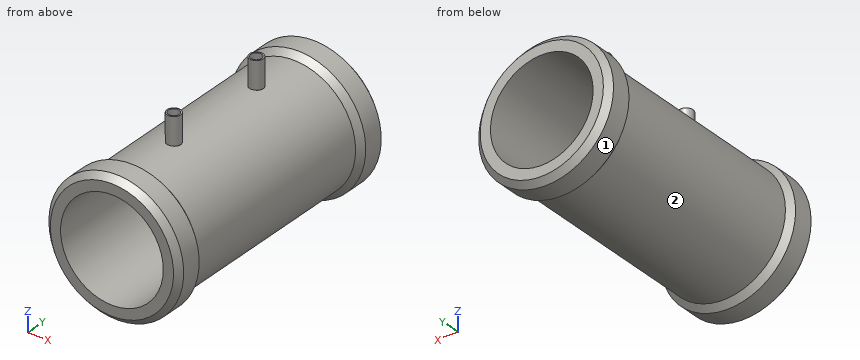
```python
from build123d import *

# Parameters (mm, degrees)
F0_R          = 45
F0_R_2        = 37.5
F1_DEPTH      = 100
F3_R          = 5
F3_R_2        = 4
F4_DEPTH      = 20
F4_DEPTH_BACK = 5


# Not quite as in the source:
# - a pattern or mirror of a feature is missing from the dataset's text; its kind, count and spacing are read off the source's solid


with BuildPart() as f1:
    # F0 (on Front) → F1 (new body, symmetric)
    with BuildSketch(Plane.XZ):
        Circle(F0_R)
        Circle(F0_R_2, mode=Mode.SUBTRACT)
    extrude(amount=F1_DEPTH, both=True)

    # F3 (on offset) → F4 (join, two sides)
    with BuildSketch(Plane.XY.offset(45)) as f4_sk:
        with Locations((0, 40)):
            Circle(F3_R)
        with Locations((0, 40)):
            Circle(F3_R_2, mode=Mode.SUBTRACT)
        with Locations((0, -40)):
            Circle(F3_R)
        with Locations((0, -40)):
            Circle(F3_R_2, mode=Mode.SUBTRACT)
    extrude(amount=F4_DEPTH)
    extrude(f4_sk.sketch, amount=-F4_DEPTH_BACK)

    # F5 (on Top) → F6 (revolve)
    with BuildSketch(Plane.XY):
        Polygon((-49.2426406871, -95.7573593129), (-45, -100), (-45, -76.5147186258), (-49.2426406871, -80.7573593129), align=None)
    f6 = revolve(axis=Axis((0, 11.0722705722, 0), (0, 1, 0)))

    # F6_copies: F6 across plane
    add(f6.mirror(Plane.ZX))


solid = f1.part
```
Model file for the job. Use its own axes, mm. Face numbers are marked on the shaded views. Coordinates: 2 decimals unless noted, no trailing zeros. Order: outer loops, then holes, each group sorted by start corner. A loop starts at its lowest first (then second) coordinate and runs counter-clockwise, first axis right, second up. Notation, with made-up numbers: M 81,-8 L 101,-8 A14 cw 101,15 Z; hole C 82.5,82.25 d11. An arc over 180 degrees is marked long. Answer as CSV lines item,"result".
(1) Band-saw the part on C-C, the plane y = 86.5. List the corners of the cut face in (x, z), then the cut area to 3 significant figures.
Geometry says:
outline,"C 0,0 d98.49; hole C 0,0 d75"
area,"3,200 mm2"
(2) Pull direction Y, two halves, no side cores. Call the marked faces 1 and 2: +Y half, -Y half, draft (parallel to the pull), parting line (faces both ways), or undercut.
Geometry says:
face 1,"draft"
face 2,"undercut"
(3) Wall check: line 1 along Y through (x, z) = (0, 59.25); line 2 along Z through (x, y) = (0, 48); line 3 along X through (y, z) = (40, 49.25). Give the ranges that are in metal, low to high.
Geometry says:
line 1,"y = -45 to -44, -36 to -35, 35 to 36, 44 to 45"
line 2,"z = -45 to -37.5, 37.5 to 45"
line 3,"x = -5 to -4, 4 to 5"
(4) Band-saw the part on A-A, the plane z = 0. List the corners of the cut face in (x, y).
Geometry says:
outline,"M -49.24,-95.76 L -45,-100 L -37.5,-100 L -37.5,100 L -45,100 L -49.24,95.76 L -49.24,80.76 L -45,76.51 L -45,-76.51 L -49.24,-80.76 Z; M 37.5,-100 L 45,-100 L 49.24,-95.76 L 49.24,-80.76 L 45,-76.51 L 45,76.51 L 49.24,80.76 L 49.24,95.76 L 45,100 L 37.5,100 Z"
(5) Flat gauge pins, fed straight in: pin 1 (5 mm diameter, centred on x = 7, y = -70.5, fed in from -Z); pin 2 (8 mm diameter, centred on y = 67, z = -4.5, fed in from -X); pin 3 (5 mm diameter, centred on y = 26, z = 26.5, fed in from -X). Where does each tip first touch, or does it go through?
Geometry says:
pin 1,"stops at z = -44.77"
pin 2,"stops at x = -45"
pin 3,"stops at x = -38.07"
(6) Band-saw the part on B-B, the plane y = 6. List the corners of the cut face in (x, z), then the cut area to 3 significant figures.
Geometry says:
outline,"C 0,0 d90; hole C 0,0 d75"
area,"1,940 mm2"
